Source: CAD feature listing. Evaluate the final solid. Frame: model axes, mm. Face numbers are marked on the shaded views. A direction names the side the tool comes from. Coordinates: 2 decimals unless noted, no trailing zeros. Order: outer loops, then holes, each group sorted by start corner. A loop starts at its lowest first (then second) coordinate and runs counter-clockwise, first axis right, second up.
Item 1: Contact query for flat-ended pins moving along their axis: P1, Ø4, axis at x = 0, z = 21.2, coming from the +Y side; P2, Ø1.7, axis at x = 20, y = -11, coming from the +Z side; P3, Ø3, axis at x = 11.5, y = 0.5, coming from the +Z side. Output: stop coordinate, or through.
Item 2: Section C-C on y = 7.22. Return the cut outline in (x, z) (3 decimals).
Item 3: Section A-A on x = -11. State how many separate pieces and enclosed holes the cut face has, then the cut area to 3 significant figures.
Item 4: Section D-D on x = 7. Return the cut outline in (y, z).
Item 5: Reachability of the marked faces 1 and 2 from +Z, -Z, +X, -X, +Y, -Y: full face, straight path, thin tool, end or side. Return the list, or none.
Item 6: Section B-B on y = -3.8. Return the cut outline in (x, z).
Item 7: Ray query, line 1 (X direction, y = -11.15, z = 14.2); line 2 (X direction, y = -10.85, z = 31.7); line 3 (X direction, y = -11.55, z = 7.2). Return the intervals inside material, ascending.
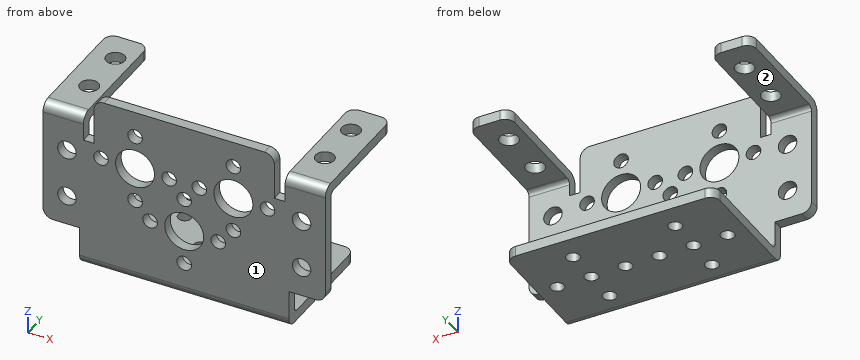
from build123d import *

# Parameters (mm, degrees)
SKETCH1_W           = 58
SKETCH1_H           = 25
BOSS_EXTRUDE1_DEPTH = 37
SKETCH2_W           = 28.8
SKETCH2_H           = 22.9
CUT_EXTRUDE1_DEPTH  = 70.923172125
CUT_EXTRUDE2_REACH  = 50.644
SKETCH3_W           = 40.6
SKETCH3_H           = 22.9
SKETCH4_W           = 7.5
SKETCH4_H           = 8
CUT_EXTRUDE3_DEPTH  = 54.244718048
CUT_EXTRUDE4_DEPTH  = 54.244718048
SKETCH8_R           = 4
SKETCH8_R_2         = 1.5
SKETCH8_R_3         = 1.9
CUT_EXTRUDE5_DEPTH  = 53.291586321
CUT_EXTRUDE6_REACH  = 47.675
SKETCH9_R           = 1.9
CUT_EXTRUDE7_REACH  = 50.644
SKETCH10_R          = 1.375
FILLET1_R           = 2
FILLET2_R           = 1


with BuildPart() as part:
    # Sketch1 → Boss-Extrude1 (new body)
    with BuildSketch(Plane.XY):
        Rectangle(SKETCH1_W, SKETCH1_H)
    extrude(amount=BOSS_EXTRUDE1_DEPTH)

    # Sketch2 → Cut-Extrude1 (cut, through all)
    with BuildSketch(Plane.ZY.offset(29)):
        with Locations((16.5, 1.05)):
            Rectangle(SKETCH2_W, SKETCH2_H)
    extrude(amount=-CUT_EXTRUDE1_DEPTH, mode=Mode.SUBTRACT)

    # Sketch3 → Cut-Extrude2 (cut, up to next)
    with BuildSketch(Plane.XY.offset(37), mode=Mode.PRIVATE) as cut_extrude2_sk1:
        with Locations((0, 1.05)):
            Rectangle(SKETCH3_W, SKETCH3_H)
    cut_extrude2_tool1 = extrude(cut_extrude2_sk1.sketch, amount=-CUT_EXTRUDE2_REACH, mode=Mode.PRIVATE) & part.part
    add(cut_extrude2_tool1.solids().sort_by_distance((0, 1.05, 37))[0], mode=Mode.SUBTRACT)

    # Sketch4 → Cut-Extrude3 (cut, through all)
    with BuildSketch(Plane.XZ.offset(12.5)):
        with Locations((-25.25, 4)):
            Rectangle(SKETCH4_W, SKETCH4_H)
        with Locations((25.25, 4)):
            Rectangle(SKETCH4_W, SKETCH4_H)
    extrude(amount=-CUT_EXTRUDE3_DEPTH, mode=Mode.SUBTRACT)

    # Sketch7 → Cut-Extrude4 (cut, through all)
    with BuildSketch(Plane.XZ.offset(12.5)):
        Polygon((-29, 37), (-18.5, 37), (-18.5, 33), (-18.5, 27.5), (-20.7, 27.5), (-20.7, 33), (-29, 33), align=None)
        Polygon((29, 37), (18.5, 37), (18.5, 33), (18.5, 27.5), (20.7, 27.5), (20.7, 33), (29, 33), align=None)
    extrude(amount=-CUT_EXTRUDE4_DEPTH, mode=Mode.SUBTRACT)

    # Sketch8 → Cut-Extrude5 (cut, through all)
    with BuildSketch(Plane(origin=(0, -10.4, 0), x_dir=(-1, 0, 0), z_dir=(0, 1, 0))):
        with Locations(Location((0, 14.2, 0), (0, 0, 90))):
            Circle(SKETCH8_R)
        with Locations(Location((7, 14.2, 0), (0, 0, 90))):
            Circle(SKETCH8_R_2)
        with Locations(Location((-7, 14.2, 0), (0, 0, 90))):
            Circle(SKETCH8_R_2)
        with Locations(Location((0, 7.2, 0), (0, 0, 90))):
            Circle(SKETCH8_R_2)
        with Locations(Location((0, 21.2, 0), (0, 0, 90))):
            Circle(SKETCH8_R_2)
        with Locations(Location((10.1, 24.7, 0), (0, 0, 90))):
            Circle(SKETCH8_R)
        with Locations(Location((17.1, 24.7, 0), (0, 0, 90))):
            Circle(SKETCH8_R_2)
        with Locations(Location((3.1, 24.7, 0), (0, 0, 90))):
            Circle(SKETCH8_R_2)
        with Locations(Location((10.1, 17.7, 0), (0, 0, 90))):
            Circle(SKETCH8_R_2)
        with Locations(Location((10.1, 31.7, 0), (0, 0, 90))):
            Circle(SKETCH8_R_2)
        with Locations(Location((-10.1, 24.7, 0), (0, 0, 90))):
            Circle(SKETCH8_R)
        with Locations(Location((-3.1, 24.7, 0), (0, 0, 90))):
            Circle(SKETCH8_R_2)
        with Locations(Location((-17.1, 24.7, 0), (0, 0, 90))):
            Circle(SKETCH8_R_2)
        with Locations(Location((-10.1, 17.7, 0), (0, 0, 90))):
            Circle(SKETCH8_R_2)
        with Locations(Location((-10.1, 31.7, 0), (0, 0, 90))):
            Circle(SKETCH8_R_2)
        with Locations(Location((24.1, 24.2, 0), (0, 0, 90))):
            Circle(SKETCH8_R_3)
        with Locations(Location((24.1, 14.1, 0), (0, 0, 90))):
            Circle(SKETCH8_R_3)
        with Locations(Location((-24.1, 14.1, 0), (0, 0, 90))):
            Circle(SKETCH8_R_3)
        with Locations(Location((-24.1, 24.2, 0), (0, 0, 90))):
            Circle(SKETCH8_R_3)
    extrude(amount=-CUT_EXTRUDE5_DEPTH, mode=Mode.SUBTRACT)

    # Sketch9 → Cut-Extrude6 (cut, up to next)
    with BuildSketch(Plane.XY.offset(33), mode=Mode.PRIVATE) as cut_extrude6_sk1:
        with Locations((-24.2, 6.2)):
            Circle(SKETCH9_R)
    cut_extrude6_tool1 = extrude(cut_extrude6_sk1.sketch, amount=-CUT_EXTRUDE6_REACH, mode=Mode.PRIVATE) & part.part
    # Sketch9 → Cut-Extrude6 (cut, up to next)
    with BuildSketch(Plane.XY.offset(33), mode=Mode.PRIVATE) as cut_extrude6_sk2:
        with Locations((-24.2, -3.8)):
            Circle(SKETCH9_R)
    cut_extrude6_tool2 = extrude(cut_extrude6_sk2.sketch, amount=-CUT_EXTRUDE6_REACH, mode=Mode.PRIVATE) & part.part
    # Sketch9 → Cut-Extrude6 (cut, up to next)
    with BuildSketch(Plane.XY.offset(33), mode=Mode.PRIVATE) as cut_extrude6_sk3:
        with Locations((24.2, 6.2)):
            Circle(SKETCH9_R)
    cut_extrude6_tool3 = extrude(cut_extrude6_sk3.sketch, amount=-CUT_EXTRUDE6_REACH, mode=Mode.PRIVATE) & part.part
    # Sketch9 → Cut-Extrude6 (cut, up to next)
    with BuildSketch(Plane.XY.offset(33), mode=Mode.PRIVATE) as cut_extrude6_sk4:
        with Locations((24.2, -3.8)):
            Circle(SKETCH9_R)
    cut_extrude6_tool4 = extrude(cut_extrude6_sk4.sketch, amount=-CUT_EXTRUDE6_REACH, mode=Mode.PRIVATE) & part.part
    add(cut_extrude6_tool1.solids().sort_by_distance((-24.2, 6.2, 33))[0], mode=Mode.SUBTRACT)
    add(cut_extrude6_tool2.solids().sort_by_distance((-24.2, -3.8, 33))[0], mode=Mode.SUBTRACT)
    add(cut_extrude6_tool3.solids().sort_by_distance((24.2, 6.2, 33))[0], mode=Mode.SUBTRACT)
    add(cut_extrude6_tool4.solids().sort_by_distance((24.2, -3.8, 33))[0], mode=Mode.SUBTRACT)

    # Sketch10 → Cut-Extrude7 (cut, up to next)
    with BuildSketch(Plane(origin=(0, 0, 0), x_dir=(-1, 0, 0), z_dir=(0, 0, -1)), mode=Mode.PRIVATE) as cut_extrude7_sk1:
        with Locations((-17.5, 0.22)):
            Circle(SKETCH10_R)
    cut_extrude7_tool1 = extrude(cut_extrude7_sk1.sketch, amount=-CUT_EXTRUDE7_REACH, mode=Mode.PRIVATE) & part.part
    # Sketch10 → Cut-Extrude7 (cut, up to next)
    with BuildSketch(Plane(origin=(0, 0, 0), x_dir=(-1, 0, 0), z_dir=(0, 0, -1)), mode=Mode.PRIVATE) as cut_extrude7_sk2:
        with Locations((-10.5, 0.22)):
            Circle(SKETCH10_R)
    cut_extrude7_tool2 = extrude(cut_extrude7_sk2.sketch, amount=-CUT_EXTRUDE7_REACH, mode=Mode.PRIVATE) & part.part
    # Sketch10 → Cut-Extrude7 (cut, up to next)
    with BuildSketch(Plane(origin=(0, 0, 0), x_dir=(-1, 0, 0), z_dir=(0, 0, -1)), mode=Mode.PRIVATE) as cut_extrude7_sk3:
        with Locations((-3.5, 0.22)):
            Circle(SKETCH10_R)
    cut_extrude7_tool3 = extrude(cut_extrude7_sk3.sketch, amount=-CUT_EXTRUDE7_REACH, mode=Mode.PRIVATE) & part.part
    # Sketch10 → Cut-Extrude7 (cut, up to next)
    with BuildSketch(Plane(origin=(0, 0, 0), x_dir=(-1, 0, 0), z_dir=(0, 0, -1)), mode=Mode.PRIVATE) as cut_extrude7_sk4:
        with Locations((3.5, 0.22)):
            Circle(SKETCH10_R)
    cut_extrude7_tool4 = extrude(cut_extrude7_sk4.sketch, amount=-CUT_EXTRUDE7_REACH, mode=Mode.PRIVATE) & part.part
    # Sketch10 → Cut-Extrude7 (cut, up to next)
    with BuildSketch(Plane(origin=(0, 0, 0), x_dir=(-1, 0, 0), z_dir=(0, 0, -1)), mode=Mode.PRIVATE) as cut_extrude7_sk5:
        with Locations((10.5, 0.22)):
            Circle(SKETCH10_R)
    cut_extrude7_tool5 = extrude(cut_extrude7_sk5.sketch, amount=-CUT_EXTRUDE7_REACH, mode=Mode.PRIVATE) & part.part
    # Sketch10 → Cut-Extrude7 (cut, up to next)
    with BuildSketch(Plane(origin=(0, 0, 0), x_dir=(-1, 0, 0), z_dir=(0, 0, -1)), mode=Mode.PRIVATE) as cut_extrude7_sk6:
        with Locations((17.5, 0.22)):
            Circle(SKETCH10_R)
    cut_extrude7_tool6 = extrude(cut_extrude7_sk6.sketch, amount=-CUT_EXTRUDE7_REACH, mode=Mode.PRIVATE) & part.part
    # Sketch10 → Cut-Extrude7 (cut, up to next)
    with BuildSketch(Plane(origin=(0, 0, 0), x_dir=(-1, 0, 0), z_dir=(0, 0, -1)), mode=Mode.PRIVATE) as cut_extrude7_sk7:
        with Locations((-10.5, 7.22)):
            Circle(SKETCH10_R)
    cut_extrude7_tool7 = extrude(cut_extrude7_sk7.sketch, amount=-CUT_EXTRUDE7_REACH, mode=Mode.PRIVATE) & part.part
    # Sketch10 → Cut-Extrude7 (cut, up to next)
    with BuildSketch(Plane(origin=(0, 0, 0), x_dir=(-1, 0, 0), z_dir=(0, 0, -1)), mode=Mode.PRIVATE) as cut_extrude7_sk8:
        with Locations((10.5, 7.22)):
            Circle(SKETCH10_R)
    cut_extrude7_tool8 = extrude(cut_extrude7_sk8.sketch, amount=-CUT_EXTRUDE7_REACH, mode=Mode.PRIVATE) & part.part
    # Sketch10 → Cut-Extrude7 (cut, up to next)
    with BuildSketch(Plane(origin=(0, 0, 0), x_dir=(-1, 0, 0), z_dir=(0, 0, -1)), mode=Mode.PRIVATE) as cut_extrude7_sk9:
        with Locations((-10.5, -6.78)):
            Circle(SKETCH10_R)
    cut_extrude7_tool9 = extrude(cut_extrude7_sk9.sketch, amount=-CUT_EXTRUDE7_REACH, mode=Mode.PRIVATE) & part.part
    # Sketch10 → Cut-Extrude7 (cut, up to next)
    with BuildSketch(Plane(origin=(0, 0, 0), x_dir=(-1, 0, 0), z_dir=(0, 0, -1)), mode=Mode.PRIVATE) as cut_extrude7_sk10:
        with Locations((10.5, -6.78)):
            Circle(SKETCH10_R)
    cut_extrude7_tool10 = extrude(cut_extrude7_sk10.sketch, amount=-CUT_EXTRUDE7_REACH, mode=Mode.PRIVATE) & part.part
    add(cut_extrude7_tool1.solids().sort_by_distance((17.5, 0.22, 0))[0], mode=Mode.SUBTRACT)
    add(cut_extrude7_tool2.solids().sort_by_distance((10.5, 0.22, 0))[0], mode=Mode.SUBTRACT)
    add(cut_extrude7_tool3.solids().sort_by_distance((3.5, 0.22, 0))[0], mode=Mode.SUBTRACT)
    add(cut_extrude7_tool4.solids().sort_by_distance((-3.5, 0.22, 0))[0], mode=Mode.SUBTRACT)
    add(cut_extrude7_tool5.solids().sort_by_distance((-10.5, 0.22, 0))[0], mode=Mode.SUBTRACT)
    add(cut_extrude7_tool6.solids().sort_by_distance((-17.5, 0.22, 0))[0], mode=Mode.SUBTRACT)
    add(cut_extrude7_tool7.solids().sort_by_distance((10.5, 7.22, 0))[0], mode=Mode.SUBTRACT)
    add(cut_extrude7_tool8.solids().sort_by_distance((-10.5, 7.22, 0))[0], mode=Mode.SUBTRACT)
    add(cut_extrude7_tool9.solids().sort_by_distance((10.5, -6.78, 0))[0], mode=Mode.SUBTRACT)
    add(cut_extrude7_tool10.solids().sort_by_distance((-10.5, -6.78, 0))[0], mode=Mode.SUBTRACT)

    # Fillet1
    fillet1_edges = [part.edges().sort_by_distance(p)[0] for p in [
        (-29, 12.5, 31.95),
        (29, 12.5, 31.95),
        (-18.5, -11.45, 37),
        (-20.7, 12.5, 31.95),
        (-24.85, -12.5, 33),
        (20.7, 12.5, 31.95),
        (18.5, -11.45, 37),
        (24.85, -12.5, 33),
        (0, -12.5, 0),
        (-29, -11.45, 8),
        (-21.5, 12.5, 1.05),
        (29, -11.45, 8),
        (21.5, 12.5, 1.05),
    ]]
    fillet(fillet1_edges, radius=FILLET1_R)

    # Fillet2
    fillet2_edges = [part.edges().sort_by_distance(p)[0] for p in [
        (-24.85, -10.4, 30.9),
        (24.85, -10.4, 30.9),
        (0, -10.4, 2.1),
    ]]
    fillet(fillet2_edges, radius=FILLET2_R)


solid = part.part
Answer list:
1. P1: stops at y = -10.4
1. P2: stops at z = 33
1. P3: stops at z = 2.1
2. outline: (-29, 30.9) - (-25.803, 30.9) - (-25.803, 33) - (-29, 33) - close; (-22.597, 30.9) - (-20.7, 30.9) - (-20.7, 33) - (-22.597, 33) - close; (-21.5, 0) - (-11.875, 0) - (-11.875, 2.1) - (-21.5, 2.1) - close; (-9.125, 0) - (9.125, 0) - (9.125, 2.1) - (-9.125, 2.1) - close; (11.875, 0) - (21.5, 0) - (21.5, 2.1) - (11.875, 2.1) - close; (20.7, 30.9) - (22.597, 30.9) - (22.597, 33) - (20.7, 33) - close; (25.803, 30.9) - (29, 30.9) - (29, 33) - (25.803, 33) - close
3. separate pieces: 7
3. enclosed holes: 0
3. area: 82.6 mm2
4. outline: (-12.5, 2) arc R2 ccw to (-10.5, 0) - (12.5, 0) - (12.5, 2.1) - (-9.4, 2.1) arc R1 cw to (-10.4, 3.1) - (-10.4, 12.7) - (-12.5, 12.7) - close; (-12.5, 15.7) - (-10.4, 15.7) - (-10.4, 22.17) - (-12.5, 22.17) - close; (-12.5, 27.23) - (-10.4, 27.23) - (-10.4, 37) - (-12.5, 37) - close
5. face 1: +Z, -Z, +X, -X, -Y
5. face 2: +X, -X, +Y
6. outline: (-29, 30.9) - (-26.1, 30.9) - (-26.1, 33) - (-29, 33) - close; (-22.3, 30.9) - (-20.7, 30.9) - (-20.7, 33) - (-22.3, 33) - close; (-21.5, 0) - (21.5, 0) - (21.5, 2.1) - (-21.5, 2.1) - close; (20.7, 30.9) - (22.3, 30.9) - (22.3, 33) - (20.7, 33) - close; (26.1, 30.9) - (29, 30.9) - (29, 33) - (26.1, 33) - close
7. line 1: x = -29 to -26, -22.2 to -8.5, -5.5 to -4, 4 to 5.5, 8.5 to 22.2, 26 to 29
7. line 2: x = -29 to -20.7, -18.5 to -11.6, -8.6 to 8.6, 11.6 to 18.5, 20.7 to 29
7. line 3: x = -21.5 to -1.5, 1.5 to 21.5
